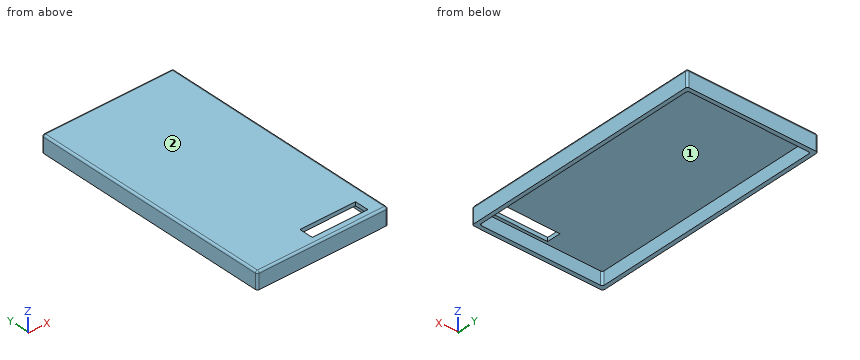
Autodesk Inventor part; units mm, degrees
ref_plane "YZ Plane" through (0, 0, 0) normal (1, 0, 0) x (0, 1, 0)
ref_plane "XZ Plane" through (0, 0, 0) normal (0, 1, 0) x (-1, 0, 0)
ref_plane "XY Plane" through (0, 0, 0) normal (0, 0, 1) x (1, 0, 0)
sketch "Sketch1" plane through (0, 0, 0) normal (0, 0, 1) x (1, 0, 0)
  line L0 (-52.798, 44.3503) -> (-52.798, -78.5857)
  line L1 (-52.798, -78.5857) -> (13.242, -78.5857)
  line L2 (13.242, -78.5857) -> (13.242, 44.3503)
  line L3 (13.242, 44.3503) -> (-52.798, 44.3503)
  point P0 (0, 0)
  dimension "d0" = 122.936
  dimension "d1" = 66.04
extrude "Extrusion1" add sketch "Sketch1" against normal blind 8.5
sketch "Sketch2" plane through (0, 0, -8.5) normal (0, 0, -1) x (-1, 0, 0)
  line L0 (-11.2347, 42.323) -> (50.7653, 42.323)
  line L1 (50.7653, 42.323) -> (50.7653, -76.5363)
  line L2 (50.7653, -76.5363) -> (-11.2347, -76.5363)
  line L3 (-11.2347, -76.5363) -> (-11.2347, 42.323)
  line L4 (52.798, 44.3503) -> (-13.242, 44.3503)
  line L5 (52.798, -78.5857) -> (52.798, 44.3503)
  line L6 (-13.242, 44.3503) -> (-13.242, -78.5857)
  line L7 (-13.242, -78.5857) -> (52.798, -78.5857)
  point P0 (0, 0)
  dimension "d16" = 62
extrude "Extrusion2" cut sketch "Sketch2" against normal blind 6.6 contours L0 L1 L2 L3
sketch "Sketch3" plane through (0, 0, -1.9) normal (0, 0, -1) x (-1, 0, 0)
  line L0 (-6.1547, -68.0123) -> (21.8453, -68.0123)
  line L1 (21.8453, -68.0123) -> (21.8453, -75.0123)
  line L2 (21.8453, -75.0123) -> (-6.1547, -75.0123)
  line L3 (-6.1547, -75.0123) -> (-6.1547, -68.0123)
  line L4 (-11.2347, -76.5363) -> (-11.2347, 42.323)
  line L5 (50.7653, -76.5363) -> (-11.2347, -76.5363)
  point P0 (0, 0)
  dimension "d10" = 5.08
  dimension "d11" = 28
  dimension "d12" = 1.524
  dimension "d13" = 7
extrude "Extrusion3" cut sketch "Sketch3" against normal blind 2.76
fillet "Fillet1" radius 1 8 edges at (11.2347, 42.323, -5.2) (13.242, 44.3503, -4.25) (-52.798, -78.5857, -4.25) (-50.7653, -76.5363, -5.2) (-50.7653, 42.323, -5.2) (-52.798, 44.3503, -4.25) (13.242, -78.5857, -4.25) (11.2347, -76.5363, -5.2)
fillet "Fillet2" radius 1 8 edges at (-52.5051, 44.0574, 0) (-52.798, -17.1177, 0) (-52.5051, -78.2928, 0) (-19.778, -78.5857, 0) (12.9491, -78.2928, 0) (13.242, -17.1177, 0) (12.9491, 44.0574, 0) (-19.778, 44.3503, 0)
properties part number "Smart Lock Box Top Correct"
Verification items for the finished model (mm, model axes). Face numbers are marked on the shaded views. Round coordinates to 2 decimals unless told otherwise and drop trailing zeros. Write each loop counter-clockwise with the first axis right and the second up, starting at its lowest first coordinate (ties: lowest second). Pieces come first, ordered by that corner, then holes.
(1) Depth check by flat-ended pin: pin 1 Ø1.5 at (x, y) = (-33, -31) entering from -Z; pin 2 Ø2 at (x, z) = (-12.5, -0.5) entering from +Y. Enter the tip coordinate at first touch or a pass-through.
Returned:
pin 1: stops at z = -1.9
pin 2: stops at y = 44.35
(2) Material ranges on line 1 (Y direction, x = -26.5, z = -2.5); line 2 (X direction, y = 6.5, z = -2); line 3 (Y direction, x = 3, z = -1.5), recorded low to high.
Returned:
line 1: y = -78.59 to -76.54, 42.32 to 44.35
line 2: x = -52.8 to -50.77, 11.23 to 13.24
line 3: y = -78.59 to -75.01, -68.01 to 44.35
(3) Section check A-A (x = -17). Enter the section's corners in (y, z).
Returned:
outline: (-78.59, -8.5) - (-76.54, -8.5) - (-76.54, -1.9) - (-75.01, -1.9) - (-75.01, 0) - (-77.59, 0) arc R1 ccw to (-78.59, -1) - close; (-68.01, -1.9) - (42.32, -1.9) - (42.32, -8.5) - (44.35, -8.5) - (44.35, -1) arc R1 ccw to (43.35, 0) - (-68.01, 0) - close
(4) Section check C-C (y = -5). Enter the section's corners in (x, z), plus the area to 3 significant figures.
Returned:
outline: (-52.8, -8.5) - (-50.77, -8.5) - (-50.77, -1.9) - (11.23, -1.9) - (11.23, -8.5) - (13.24, -8.5) - (13.24, -1) arc R1 ccw to (12.24, 0) - (-51.8, 0) arc R1 ccw to (-52.8, -1) - close
area: 152 mm2
(5) Section check B-B (z = -7). Enter the section's corners in (x, y), plus the area to 3 significant figures.
Returned:
outline: (-52.8, -77.59) arc R1 ccw to (-51.8, -78.59) - (12.24, -78.59) arc R1 ccw to (13.24, -77.59) - (13.24, 43.35) arc R1 ccw to (12.24, 44.35) - (-51.8, 44.35) arc R1 ccw to (-52.8, 43.35) - close; hole (-50.77, -75.54) arc R1 ccw to (-49.77, -76.54) - (10.23, -76.54) arc R1 ccw to (11.23, -75.54) - (11.23, 41.32) arc R1 ccw to (10.23, 42.32) - (-49.77, 42.32) arc R1 ccw to (-50.77, 41.32) - close
area: 749 mm2
(6) Mould release check, pull along Y, two halves, no side actions. Record for the marked faces 1 and 2: pulls with the +Y half, pulls with the -Y half, needs draft (parallel to the pull), parting line crosses it, or undercut.
Returned:
face 1: undercut
face 2: needs draft
(7) Section check D-D (x = -46). Enter the section's corners in (y, z).
Returned:
outline: (-78.59, -8.5) - (-76.54, -8.5) - (-76.54, -1.9) - (42.32, -1.9) - (42.32, -8.5) - (44.35, -8.5) - (44.35, -1) arc R1 ccw to (43.35, 0) - (-77.59, 0) arc R1 ccw to (-78.59, -1) - close
